Part model, mm, in its own coordinate system. Round coordinates to 2 decimals unless told otherwise and drop trailing zeros. Loops run counter-clockwise (first coordinate to the right, second up) from the corner with the lowest first, then second, coordinate; pieces in that order, holes last. Notation, with made-up numbers: M -16,26.25 L 42,26.25 A24 cw 42,54.25 Z; hole C 16.25,51 d8. An arc over 180 degrees is marked long. Write each question's results on one line, items separated by ' | '.
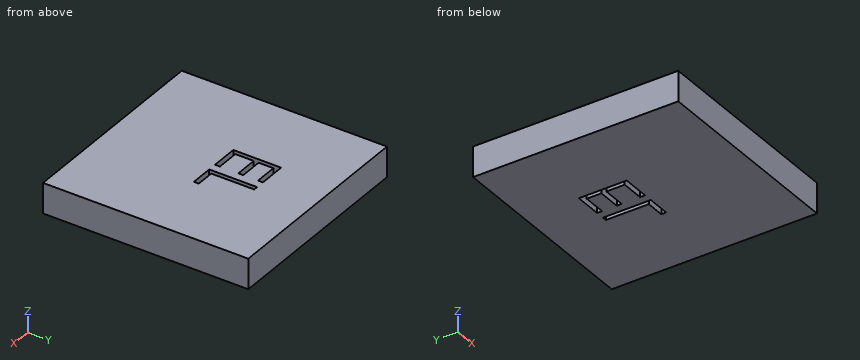
from build123d import *

# Parameters (mm, degrees)
SKETCH1_W           = 15
SKETCH1_H           = 15
BOSS_EXTRUDE1_DEPTH = 2.21


with BuildPart() as part:
    # Sketch1 → Boss-Extrude1 (new body)
    with BuildSketch(Plane.XY):
        with Locations((7.5, 7.5)):
            Rectangle(SKETCH1_W, SKETCH1_H)
        Polygon((5.525641026, 11), (7.5, 11), (7.5, 10.641025641), (5.83974359, 10.641025641), (5.83974359, 9.564102564), (7.5, 9.564102564), (7.5, 9.205128205), (5.83974359, 9.205128205), (5.83974359, 7.858974359), (7.5, 7.858974359), (7.5, 7.5), (5.525641026, 7.5), align=None, mode=Mode.SUBTRACT)
        Polygon((8.128205128, 11), (8.442307692, 11), (8.442307692, 7.858974359), (9.788461538, 7.858974359), (9.788461538, 7.5), (8.128205128, 7.5), align=None, mode=Mode.SUBTRACT)
    extrude(amount=BOSS_EXTRUDE1_DEPTH)


solid = part.part
Item 1: Band-saw the part on A-A on y = 8.75. Give the cut face in (x, z).
Filled sheet:
outline: M 0,0 L 5.53,0 L 5.53,2.21 L 0,2.21 Z; M 5.84,0 L 8.13,0 L 8.13,2.21 L 5.84,2.21 Z; M 8.44,0 L 15,0 L 15,2.21 L 8.44,2.21 Z
Item 2: Band-saw the part on D-D on z = 0.8. Give the cut face in (x, y), and give its area (3 significant figures).
Filled sheet:
outline: M 0,0 L 15,0 L 15,15 L 0,15 Z; hole M 5.53,7.5 L 7.5,7.5 L 7.5,7.86 L 5.84,7.86 L 5.84,9.21 L 7.5,9.21 L 7.5,9.56 L 5.84,9.56 L 5.84,10.64 L 7.5,10.64 L 7.5,11 L 5.53,11 Z; hole M 8.13,7.5 L 9.79,7.5 L 9.79,7.86 L 8.44,7.86 L 8.44,11 L 8.13,11 Z | area: 221 mm^2
Item 3: Band-saw the part on B-B on x = 8.75. Give the cut face in (y, z), and give its area (3 significant figures).
Filled sheet:
outline: M 0,0 L 7.5,0 L 7.5,2.21 L 0,2.21 Z; M 7.86,0 L 15,0 L 15,2.21 L 7.86,2.21 Z | area: 32.4 mm^2
Item 4: Band-saw the part on C-C on x = 6.25. Give the cut face in (y, z), and give its area (3 significant figures).
Filled sheet:
outline: M 0,0 L 7.5,0 L 7.5,2.21 L 0,2.21 Z; M 7.86,0 L 9.21,0 L 9.21,2.21 L 7.86,2.21 Z; M 9.56,0 L 10.64,0 L 10.64,2.21 L 9.56,2.21 Z; M 11,0 L 15,0 L 15,2.21 L 11,2.21 Z | area: 30.8 mm^2
Item 5: Wall check: L1, parallel to X at y = 8.5, z = 0.4; L2, parallel to Y at x = 6.25, z = 0.9; L3, parallel to Y at x = 5.75, z = 2. Give the ranges that are in metal, low to high.
Filled sheet:
L1: 0 to 5.53, 5.84 to 8.13, 8.44 to 15 | L2: 0 to 7.5, 7.86 to 9.21, 9.56 to 10.64, 11 to 15 | L3: 0 to 7.5, 11 to 15
